from build123d import *

# Parameters (mm, degrees)
DODANIE_WYCI_GNI_CIE1_DEPTH = 6
SZKIC2_R                    = 2.05
WYTNIJ_WYCI_GNI_CIE1_DEPTH  = 6
SZKIC3_R                    = 1.55
WYTNIJ_WYCI_GNI_CIE2_DEPTH  = 6


with BuildPart() as part:
    # Szkic1 → Dodanie-wyciągnięcie1 (new body)
    with BuildSketch(Plane.XY):
        with BuildLine():
            Line((135.201456632, 17.703969636), (27.201456632, 17.703969636))
            ThreePointArc((27.201456632, 17.703969636), (21.201456632, 11.703969636), (27.201456632, 5.703969636))
            Line((27.201456632, 5.703969636), (135.201456632, 5.703969636))
            ThreePointArc((135.201456632, 5.703969636), (141.201456632, 11.703969636), (135.201456632, 17.703969636))
        make_face()
    extrude(amount=DODANIE_WYCI_GNI_CIE1_DEPTH)

    # Szkic2 → Wytnij-wyciągnięcie1 (cut)
    with BuildSketch(Plane.XY.offset(6)):
        with Locations((135.201456632, 11.703969636)):
            Circle(SZKIC2_R)
        with Locations((27.201456632, 11.703969636)):
            Circle(SZKIC2_R)
    extrude(amount=-WYTNIJ_WYCI_GNI_CIE1_DEPTH, mode=Mode.SUBTRACT)

    # Szkic3 → Wytnij-wyciągnięcie2 (cut)
    with BuildSketch(Plane.XY.offset(6)):
        with Locations((53.201456632, 11.703969636)):
            Circle(SZKIC3_R)
        with Locations((81.201456632, 11.703969636)):
            Circle(SZKIC3_R)
        with Locations((109.201456632, 11.703969636)):
            Circle(SZKIC3_R)
    extrude(amount=-WYTNIJ_WYCI_GNI_CIE2_DEPTH, mode=Mode.SUBTRACT)


solid = part.part
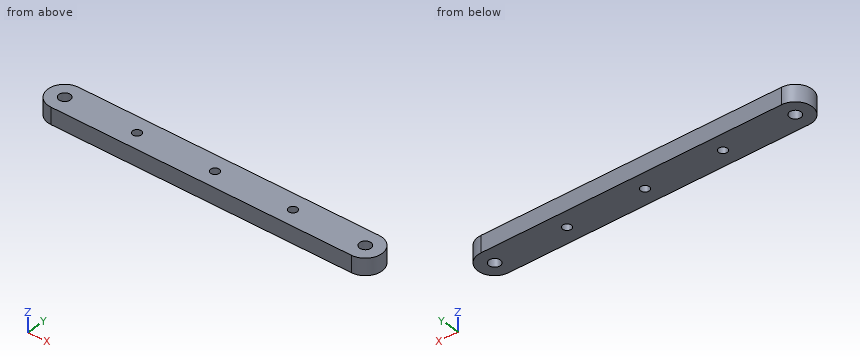
Verification items for the finished model (mm, model axes). Coordinates: 2 decimals unless noted, no trailing zeros. Loops run counter-clockwise (first coordinate to the right, second up) from the corner with the lowest first, then second, coordinate; pieces in that order, holes last. Notation, with made-up numbers: (70, 30) -> (103, 30) arc R21 ccw to (103, 43) -> close; hole circle Ø9 at (0, -19.5). An arc over 180 degrees is marked (long way). Write each question's results on one line, items separated by ' | '.
Item 1: Material ranges on L1, parallel to X at y = 10.5, z = 1.8; L2, parallel to X at y = 12.5, z = 2.9; L3, parallel to X at y = 6.75, z = 2, recorded low to high.
Found:
L1: x = 21.32 to 25.54, 28.86 to 52.23, 54.18 to 80.23, 82.18 to 108.23, 110.18 to 133.54, 136.86 to 141.08 | L2: x = 21.25 to 25.31, 29.09 to 51.87, 54.53 to 79.87, 82.53 to 107.87, 110.53 to 133.31, 137.09 to 141.15 | L3: x = 23.82 to 138.59
Item 2: Section check C-C, the plane y = 7. Enter the section's corners in (x, z), plus the area to 3 significant figures.
Found:
outline: (23.48, 0) -> (138.93, 0) -> (138.93, 6) -> (23.48, 6) -> close | area: 693 mm2
Item 3: Section check B-B, the plane x = 81. Enter the section's corners in (y, z).
Found:
outline: (5.7, 0) -> (10.17, 0) -> (10.17, 6) -> (5.7, 6) -> close; (13.24, 0) -> (17.7, 0) -> (17.7, 6) -> (13.24, 6) -> close
Item 4: Section check D-D, the plane y = 15.75. Enter the section's corners in (x, z).
Found:
outline: (22.77, 0) -> (139.63, 0) -> (139.63, 6) -> (22.77, 6) -> close
Item 5: Gauge pin test, flat ends, axial feed: pin 1 (5.5 mm diameter, centred on x = 27.2, y = 11.7, fed in from -Z); pin 2 (2 mm diameter, centred on y = 10, z = 5.5, fed in from +X); pin 3 (1.5 mm diameter, centred on y = 13, z = 5, fed in from -X); pin 4 (1.5 mm diameter, centred on y = 9, z = 2, fed in from -X). Record the tip position at first contact, or that the pin passes through.
Found:
pin 1: stops at z = 0 | pin 2: stops at x = 141.16 | pin 3: stops at x = 21.23 | pin 4: stops at x = 21.53
Item 6: Section check A-A, the plane z = 0.9. Enter the section's corners in (x, y), plus the area to 3 significant figures.
Found:
outline: (27.2, 5.7) -> (135.2, 5.7) arc R6 ccw to (135.2, 17.7) -> (27.2, 17.7) arc R6 ccw to start; hole circle Ø4.1 at (27.2, 11.7); hole circle Ø3.1 at (53.2, 11.7); hole circle Ø3.1 at (81.2, 11.7); hole circle Ø3.1 at (109.2, 11.7); hole circle Ø4.1 at (135.2, 11.7) | area: 1,360 mm2
